Check sheet for the drawn part. Datum: minimum x, y, z corner. Units: mm. Coordinates: 2 decimals unless noted, no trailing zeros. Order: outer loops, then holes, each group sorted by start corner. A loop starts at its lowest first (then second) coordinate and runs counter-clockwise, first axis right, second up. Notation, with made-up numbers: (79.25, -33) - (135.25, -33) arc R24 cw to (135.25, -17) - close; hole circle Ø7 at (22.25, -15). An arc over 180 degrees is marked (long way). Answer as CSV lines item,"result". Start each with the question number.
1. Section check A-A (y = 20). Record the cut outline in (x, z), and give its area (3 significant figures).
2. Section check D-D (y = 60). Record the cut outline in (x, z).
3. Material ranges on L1, parallel to Y at x = 22, z = 16.25; L2, parallel to Y at x = 135, z = 10.5; L3, parallel to Z at x = 90, y = 34, recorded low to high. Write a range as [from, to].
4. Section check C-C (z = 2.25). Record the cut outline in (x, y), and give its area (3 significant figures).
5. Go/stop test with flat-tipped pins: pin 1 (2 mm diameter, centred on y = 41, z = 15.5, fed in from -X); pin 2 (5.5 mm diameter, centred on x = 9, z = 17.5, fed in from +Y); pin 3 (5.5 mm diameter, centred on x = 19, z = 17, fed in from -Y); pin 4 (1.5 mm diameter, centred on y = 73, z = 16.5, fed in from +X). Record where each tip stops, or that it passes through.
6. Mould release check, pull along X, two halves, no side actions. Record for the marked faces 1, 2 and 3: pulls with the +X half, pulls with the -X half, needs draft (parallel to the pull), parting line crosses it, or undercut.
7. Section check B-B (x = 135). Record the cut outline in (y, z).
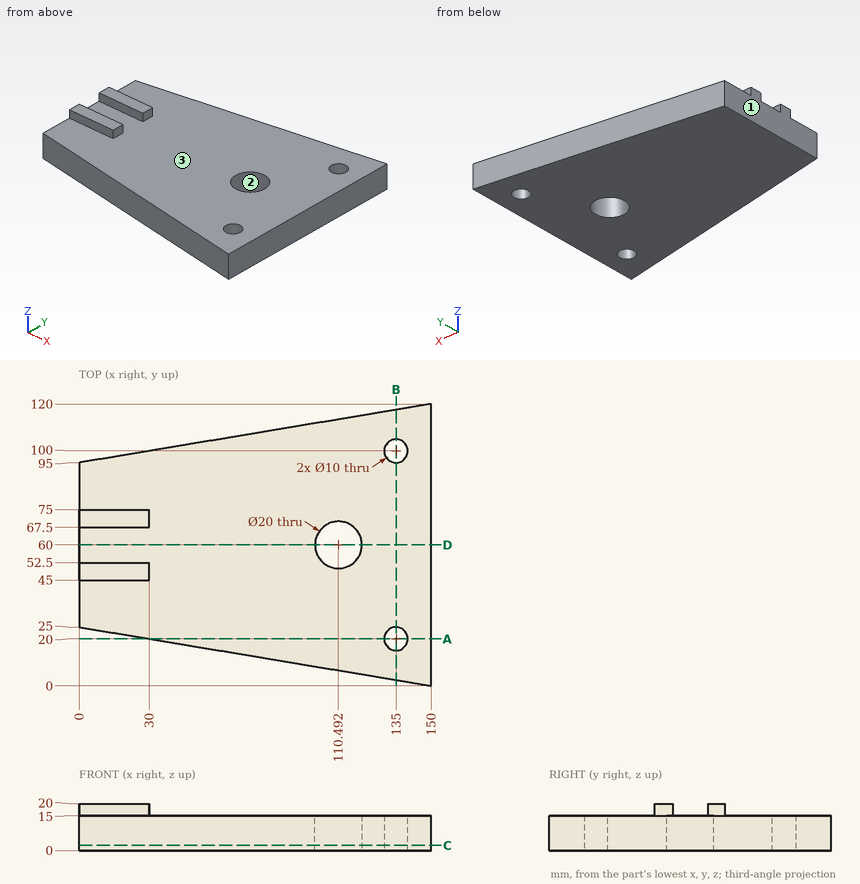
Evaluation:
1,outline,"(30, 0) - (130, 0) - (130, 15) - (30, 15) - close; (140, 0) - (150, 0) - (150, 15) - (140, 15) - close"
1,area,"1,650 mm²"
2,outline,"(0, 0) - (100.49, 0) - (100.49, 15) - (0, 15) - close; (120.49, 0) - (150, 0) - (150, 15) - (120.49, 15) - close"
3,L1,"y = [45, 52.5], [67.5, 75]"
3,L2,"y = [2.5, 15], [25, 95], [105, 117.5]"
3,L3,"z = [0, 15]"
4,outline,"(0, 25) - (150, 0) - (150, 120) - (0, 95) - close; hole circle Ø20 at (110.49, 60); hole circle Ø10 at (135, 20); hole circle Ø10 at (135, 100)"
4,area,"13,800 mm²"
5,pin 1,"stops at x = 0"
5,pin 2,"stops at y = 96.69"
5,pin 3,"stops at y = 21.52"
5,pin 4,"stops at x = 30"
6,face 1,"pulls with the -X half"
6,face 2,"undercut"
6,face 3,"needs draft"
7,outline,"(2.5, 0) - (15, 0) - (15, 15) - (2.5, 15) - close; (25, 0) - (95, 0) - (95, 15) - (25, 15) - close; (105, 0) - (117.5, 0) - (117.5, 15) - (105, 15) - close"
